For this review, take the finished solid that the model builds, in its own axes (mm). Face numbers are marked on the shaded views. A direction names the side the tool comes from. Coordinates: 2 decimals unless noted, no trailing zeros. Order: outer loops, then holes, each group sorted by start corner. A loop starts at its lowest first (then second) coordinate and runs counter-clockwise, first axis right, second up. Notation, with made-up numbers: (28, 55) -> (62, 55) arc R16 cw to (62, 63) -> close; hole circle Ø8 at (69.5, -21.5). An arc over 180 degrees is marked (long way). Answer as a JSON object with one key per item and string values. Group by question number.
1) Draft analysis for pull direction X (two halves, no side actions). For the marked faces 1, 2, 3 and 4, state which applies: +X half, -X half, draft (parallel to the pull), parting line (faces both ways), or undercut.
2) Wall thickness on L1, parallel to Z at x = -23.8, y = 1; L2, parallel to X at y = -7, z = 1.5; L3, parallel to Y at x = -7.5, z = 2.75: over which ranges is each line inside the solid? List them lowest first.
3) Add section D-D, the plane x = -19. Write out the cut boundary in (y, z), then the cut area to 3 significant figures.
4) For pin 1 (4 mm diameter, centred on x = -15.5, y = -5, fed in from -Z); pin 2 (0.8 mm diameter, centred on y = 1.5, z = 28, fed in from -X); pin 3 (0.8 mm diameter, centred on x = -24.5, y = 0.5, fed in from +Z); pin 4 (1.8 mm diameter, centred on y = 1, z = 2.5, fed in from -X), all flat-tipped, find the tip position at first contact; note any pin that passes through.
5) Add section B-B, the plane x = 0. Write out the cut boundary in (y, z).
6) Machinability: for the marked faces 5, 6 and 7, which of the approach directions +Z, -Z, +X, -X, +Y, -Y give a long, thin tool a straight path to every point of the face, cutting with its end or side? Answer none if there is none.
7) Add section A-A, the plane z = 2.5. Write out the cut boundary in (x, y), then the cut area to 3 significant figures.
8) Add section C-C, the plane y = -4.5. Write out the cut boundary in (x, z), then the cut area to 3 significant figures.
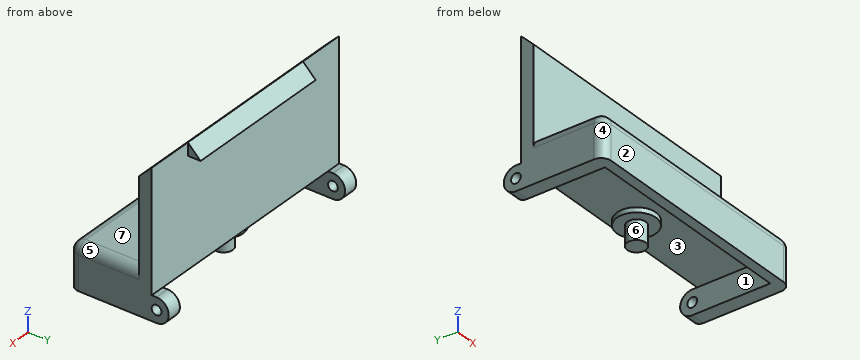
from build123d import *

# Parameters (mm, degrees)
PAD003_DEPTH    = 25.25
SKETCH008_W     = 25
SKETCH008_H     = 44.5
POCKET_DEPTH    = 5
SKETCH009_R     = 4
PAD004_DEPTH    = 1
SKETCH010_R     = 1.9
PAD005_DEPTH    = 4
POCKET001_DEPTH = 5
SKETCH012_R     = 1
POCKET002_DEPTH = 50.501
FILLET_R        = 2


with BuildPart() as part:
    # Sketch003 → Pad003 (new body, symmetric)
    with BuildSketch(Plane.YZ):
        with BuildLine():
            Line((-2.6, 27.03), (-2.6, 9))
            Line((-2.6, 9), (-17, 9))
            Line((-17, 9), (-17, 0))
            Line((-17, 0), (1, 0))
            ThreePointArc((1, 0), (3.5, 2.5), (1, 5))
            Line((0, 5), (1, 5))
            Line((0, 5), (0, 27.03))
            Line((0, 27.03), (2.6, 27.03))
            Line((2.6, 27.03), (0, 29.63))
            Line((0, 29.63), (-2.6, 27.03))
        make_face()
    extrude(amount=PAD003_DEPTH, both=True)

    # Sketch008 (on Face8 of Pad003) → Pocket (cut)
    with BuildSketch(Plane.YX):
        with Locations((-2.5, 0)):
            Rectangle(SKETCH008_W, SKETCH008_H)
    extrude(amount=-POCKET_DEPTH, mode=Mode.SUBTRACT)

    # Sketch009 (on Face3 of Pocket) → Pad004 (join)
    with BuildSketch(Plane.YX.offset(-5)):
        with Locations((-4.5, 0)):
            Circle(SKETCH009_R)
    extrude(amount=PAD004_DEPTH)

    # Sketch010 (on Face20 of Pad004) → Pad005 (join)
    with BuildSketch(Plane.YX.offset(-4)):
        with Locations((-4.5, 0)):
            Circle(SKETCH010_R)
    extrude(amount=PAD005_DEPTH)

    # Sketch011 (on Face5 of Pad005) → Pocket001 (cut)
    with BuildSketch(Plane.YX.offset(-27.03)):
        Polygon((0, 15.5), (5, 15.5), (5, -15.5), (0, -15.5), (0, -30), (22, -30), (22, 30), (0, 30), align=None)
    extrude(amount=-POCKET001_DEPTH, mode=Mode.SUBTRACT)

    # Sketch012 (on Face9 of Pocket001) → Pocket002 (cut, through all)
    with BuildSketch(Plane.YZ.offset(25.25)):
        with Locations((1, 2.5)):
            Circle(SKETCH012_R)
    extrude(amount=-POCKET002_DEPTH, mode=Mode.SUBTRACT)

    # Fillet
    fillet_edges = [part.edges().sort_by_distance(p)[0] for p in [
        (0, -17, 9),
        (25.25, -17, 4.5),
        (25.25, -9.8, 9),
        (-25.25, -17, 4.5),
        (-25.25, -9.8, 9),
    ]]
    fillet(fillet_edges, radius=FILLET_R)


solid = part.part
Output values:
{
 "1": {"face 1": "undercut", "face 2": "draft", "face 3": "undercut", "face 4": "-X half"},
 "2": {"L1": "z = 0 to 1.5, 3.5 to 5", "L2": "x = -25.25 to -22.25, 22.25 to 25.25", "L3": "y = -17 to -15"},
 "3": {"outline": "(-17, 0) -> (-15, 0) -> (-15, 5) -> (0, 5) -> (0, 29.63) -> (-2.6, 27.03) -> (-2.6, 9) -> (-15, 9) arc R2 ccw to (-17, 7) -> close", "area": "127 mm²"},
 "4": {"pin 1": "stops at z = 5", "pin 2": "stops at x = -15.5", "pin 3": "stops at z = 5", "pin 4": "passes through"},
 "5": {"outline": "(-17, 0) -> (-15, 0) -> (-15, 5) -> (-8.5, 5) -> (-8.5, 4) -> (-6.4, 4) -> (-6.4, 0) -> (-2.6, 0) -> (-2.6, 4) -> (-0.5, 4) -> (-0.5, 5) -> (0, 5) -> (0, 27.03) -> (2.6, 27.03) -> (0, 29.63) -> (-2.6, 27.03) -> (-2.6, 9) -> (-15, 9) arc R2 ccw to (-17, 7) -> close"},
 "6": {"face 5": "+Z, +X, -Y", "face 6": "-Z", "face 7": "+Z, +X, -X, -Y"},
 "7": {"outline": "(-25.25, -15) arc R2 ccw to (-23.25, -17) -> (23.25, -17) arc R2 ccw to (25.25, -15) -> (25.25, 0) -> (22.25, 0) -> (22.25, -15) -> (-22.25, -15) -> (-22.25, 0) -> (-25.25, 0) -> close; (-25.25, 2) -> (-22.25, 2) -> (-22.25, 3.5) -> (-25.25, 3.5) -> close; circle Ø3.8 at (0, -4.5); (22.25, 2) -> (25.25, 2) -> (25.25, 3.5) -> (22.25, 3.5) -> close", "area": "210 mm²"},
 "8": {"outline": "(-25.25, 0) -> (-22.25, 0) -> (-22.25, 5) -> (-4, 5) -> (-4, 4) -> (-1.9, 4) -> (-1.9, 0) -> (1.9, 0) -> (1.9, 4) -> (4, 4) -> (4, 5) -> (22.25, 5) -> (22.25, 0) -> (25.25, 0) -> (25.25, 7) arc R2 ccw to (23.25, 9) -> (-23.25, 9) arc R2 ccw to (-25.25, 7) -> close", "area": "253 mm²"}
}
